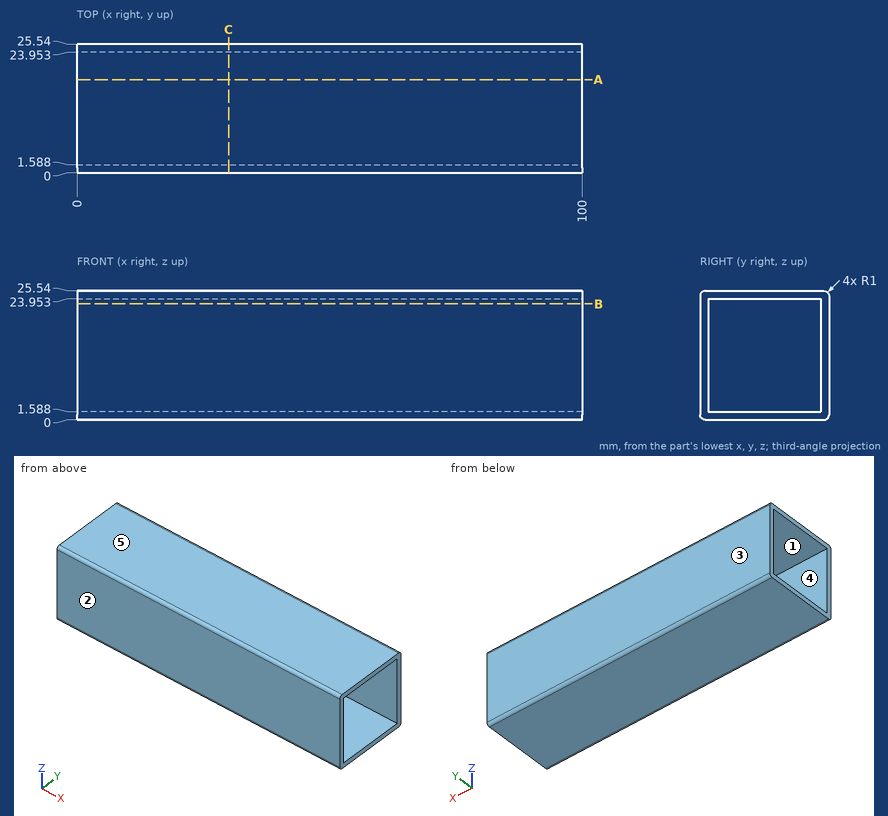
Design review of the part shown in the three views and the two pictorial views. Dimensions are in mm from the part's minimum x, y and z. A direction names the side the tool comes from. Give positions to 0.01 mm unless a question says otherwise; leave off trailing zeros. Loops run counter-clockwise (first coordinate to the right, second up) from the corner with the lowest first, then second, coordinate; pieces in that order, holes last. Notation, with made-up numbers: M 24.5,0 L 51.5,0 A18 ccw 51.5,12 Z; hole C 69.25,-3 d2. An arc over 180 degrees is marked long. Write item = value, one per line.
Q1. We need section C-C (x = 30). Give the boundary of the cut face in (y, z), plus the area to 3 significant figures.
Output values:
outline = M 0,1 A1 ccw 1,0 L 24.54,0 A1 ccw 25.54,1 L 25.54,24.54 A1 ccw 24.54,25.54 L 1,25.54 A1 ccw 0,24.54 Z; hole M 1.59,1.59 L 23.95,1.59 L 23.95,23.95 L 1.59,23.95 Z
area = 151 mm^2
Q2. For the marked faces 1 and 2, list the 3-axis set-ups (+Z, -Z, +X, -X, +Y, -Y) from which the entire face can be reached by the end or side of a thin tool; tool diameter is ignored.
Output values:
face_1 = +X, -X
face_2 = +Z, -Z, +X, -X, -Y
Q3. We need section A-A (y = 18.5). Give the boundary of the cut face in (x, z).
Output values:
outline = M 0,0 L 100,0 L 100,1.59 L 0,1.59 Z; M 0,23.95 L 100,23.95 L 100,25.54 L 0,25.54 Z
Q4. Draft analysis for pull direction Y (two halves, no side actions). For the marked faces 3, 4 and 5, state which applies: +Y half, -Y half, draft (parallel to the pull), parting line (faces both ways), or undercut.
Output values:
face_3 = +Y half
face_4 = undercut
face_5 = draft
Q5. To check wall thickness, follow line 1 (Z direction, x = 83.5, y = 14.5). State the ranges of the line that lie inside material, in increasing order. Write a range as [from, to].
Output values:
line_1 = [0, 1.59], [23.95, 25.54]
